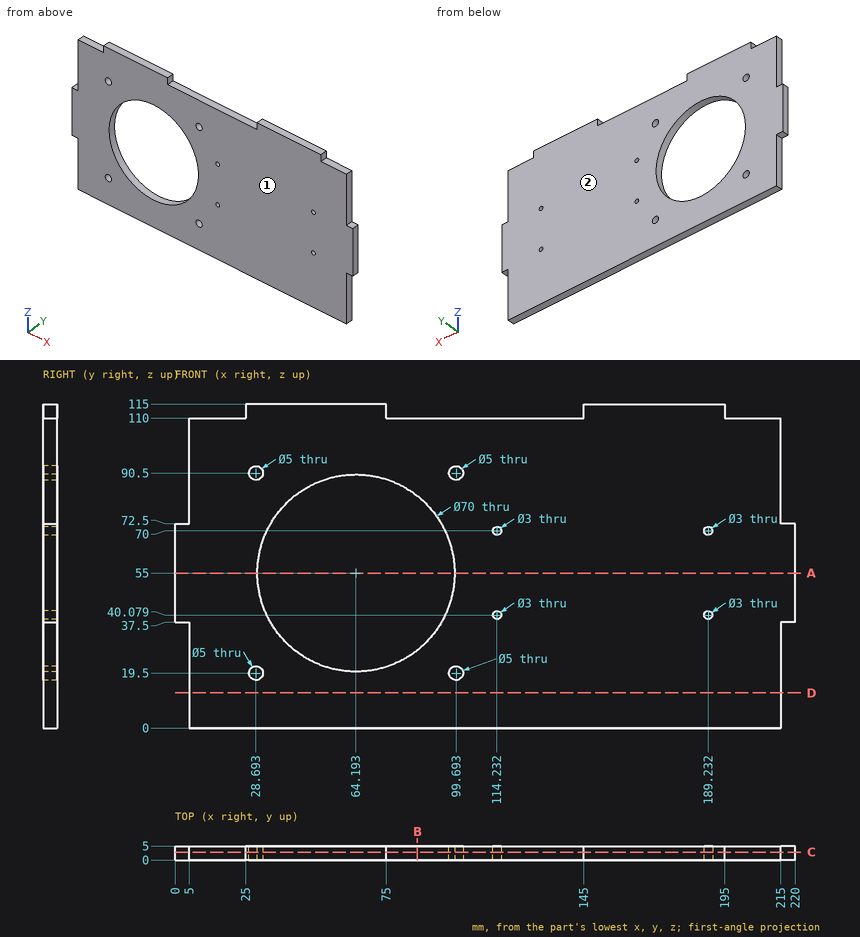
Here's the drawing with two shaded views (mm, measured from the low corner). I have some questions. Coordinates: 2 decimals unless noted, no trailing zeros. Loops run counter-clockwise (first coordinate to the right, second up) from the corner with the lowest first, then second, coordinate; pieces in that order, holes last. Notation, with made-up numbers: M 64,19.25 L 116,19.25 A33 ccw 116,58.25 Z; hole C -30.75,31.5 d8. An arc over 180 degrees is marked long. Answer as CSV lines item,"result". Start each with the question number.
1. If I drill on probe 1 along Z at (x, y) = (100, 3.65); probe 2 along X at (y, z) = (1.7, 40) (1 decimal); probe 3 along Z at (x, y) = (188, 3.6) (1 decimal), over which ranges is the centre line in solid material (lowest first)? Write a range as [from, to].
2. Thinking about a two-plate mould opening in Y: for the marked faces 1 and 2, which applies, +Y half, -Y half, draft (parallel to the pull), parting line (faces both ways), or undercut?
3. For pin 1 Ø1.5 at (y, z) = (3.5, 15.5) entering from -X; pin 2 Ø1.5 at (x, y) = (3, 3) entering from +Z; pin 3 Ø2.5 at (y, z) = (2.5, 111.5) entering from -X, each with a flat end and sliding along its axis, tell me the tip position at first contact or that it passes through.
4. Suppose I cut it at A-A, the plane z = 55. List the corners of the cut face in (x, y) for me.
5. Suppose I cut it at D-D, the plane z = 12.5. List the corners of the cut face in (x, y) for me, plus the area to 3 significant figures.
6. Suppose I cut it at B-B, the plane x = 86. List the corners of the cut face in (y, z) for me, plus the area to 3 significant figures.
7. Suppose I cut it at C-C, the plane y = 2.8. Count the separate pieces of the cut face and the enclosed holes in it, plus the area to 3 significant figures.
Output:
1,probe 1,"z = [0, 17.02], [21.98, 88.02], [92.98, 110]"
1,probe 2,"x = [0, 32.6], [95.8, 112.7], [115.7, 187.7], [190.7, 220]"
1,probe 3,"z = [0, 39.2], [40.9, 69.1], [70.9, 115]"
2,face 1,"-Y half"
2,face 2,"+Y half"
3,pin 1,"stops at x = 5"
3,pin 2,"stops at z = 72.5"
3,pin 3,"stops at x = 25"
4,outline,"M 0,0 L 29.19,0 L 29.19,5 L 0,5 Z; M 99.19,0 L 220,0 L 220,5 L 99.19,5 Z"
5,outline,"M 5,0 L 215,0 L 215,5 L 5,5 Z"
5,area,"1,050 mm^2"
6,outline,"M 0,0 L 5,0 L 5,27.62 L 0,27.62 Z; M 0,82.38 L 5,82.38 L 5,110 L 0,110 Z"
6,area,"276 mm^2"
7,separate pieces,"1"
7,enclosed holes,"9"
7,area,"20,000 mm^2"
